Design review of the part built by this model. Coordinates are the model's own, in mm. A direction names the side the tool comes from. Coordinates: 2 decimals unless noted, no trailing zeros. Loops run counter-clockwise (first coordinate to the right, second up) from the corner with the lowest first, then second, coordinate; pieces in that order, holes last. Notation, with made-up numbers: (-16.5, 48.5) -> (20.5, 48.5) arc R29 cw to (20.5, 78.5) -> close; hole circle Ø5 at (-17, 28.25). An arc over 180 degrees is marked (long way). One line per item, written item: value. Start each with the question number.
1. Add section A-A on x = 38. Write out the cut boundary in (y, z), plus the area to 3 significant figures.
2. Add section C-C on x = 82.5. Write out the cut boundary in (y, z), plus the area to 3 significant figures.
3. Draft analysis for pull direction X (two halves, no side actions). For faces 5 (the flat face through (138.7, 24, 1)), 6 (the flat face through (46.24, 36, 2)), 7 (the flat face through (67, 24, 3)), state which applies: pulls with the +X half, pulls with the -X half, needs draft (parallel to the pull), parting line crosses it, or undercut.
4. For probe 1 along X at (y, z) = (13, 2.75); probe 2 along Y at (x, z) = (46, 0.25); probe 3 along X at (y, z) = (9, 2.35), list the stretches that pass through material, from the lowest coordinate up.
5. Insertion check: pin 1 (1.5 mm diameter, centred on x = 36, z = 1, fed in from -Y); pin 2 (0.9 mm diameter, centred on y = 13, z = 1.5, fed in from -X). Each pin has a flat end and moves straight along its axis. Give the tip position at first contact, or say it passes through.
6. Machinability: for faces 1 (the flat face through (100, 37.459, 2)), 2 (the flat face through (69, 8.959, 1)), 3 (the flat face through (-1, 33.959, 1)), 4 (the flat face through (-3, 27, 1)), which of the approach directions +Z, -Z, +X, -X, +Y, -Y give a long, thin tool a straight path to every point of the face, cutting with its end or side? Answer none if there is none.
7. Add section B-B on z = 0.9. Write out the cut boundary in (x, y), plus the area to 3 significant figures.
```python
from build123d import *

# Parameters (mm, degrees)
BOSS_EXTRUDE1_DEPTH = 3
SKETCH2_W           = 15
SKETCH2_H           = 3
CUT_EXTRUDE1_DEPTH  = 4


with BuildPart() as part:
    # Sketch1 → Boss-Extrude1 (new body)
    with BuildSketch(Plane.XY):
        with BuildLine():
            Line((138.7, 8.95909513), (138.7, 38.95909513))
            Line((138.7, 38.95909513), (0, 38.95909513))
            Line((0, 38.95909513), (0, 33.95909513))
            Line((0, 33.95909513), (-3, 33.95909513))
            Line((-3, 33.95909513), (-3, 18.95909513))
            Line((-3, 18.95909513), (0, 18.95909513))
            Line((0, 18.95909513), (0, 8.95909513))
            ThreePointArc((0, 8.95909513), (10, -1.04090487), (20, 8.95909513))
            Line((20, 8.95909513), (118.7, 8.95909513))
            ThreePointArc((118.7, 8.95909513), (128.7, -1.04090487), (138.7, 8.95909513))
        make_face()
    extrude(amount=BOSS_EXTRUDE1_DEPTH)

    # Sketch2 → Cut-Extrude1 (cut, through all)
    with BuildSketch(Plane.XY.offset(3)):
        with Locations((38.74, 35.95909513)):
            Rectangle(SKETCH2_W, SKETCH2_H)
        with Locations((99.97, 35.95909513)):
            Rectangle(SKETCH2_W, SKETCH2_H)
        with Locations((38.74, 11.95909513)):
            Rectangle(SKETCH2_W, SKETCH2_H)
        with Locations((99.97, 11.95909513)):
            Rectangle(SKETCH2_W, SKETCH2_H)
    extrude(amount=-CUT_EXTRUDE1_DEPTH, mode=Mode.SUBTRACT)


solid = part.part
```
Worked answers:
1. outline: (8.96, 0) -> (10.46, 0) -> (10.46, 3) -> (8.96, 3) -> close; (13.46, 0) -> (34.46, 0) -> (34.46, 3) -> (13.46, 3) -> close; (37.46, 0) -> (38.96, 0) -> (38.96, 3) -> (37.46, 3) -> close
1. area: 72.0 mm²
2. outline: (8.96, 0) -> (38.96, 0) -> (38.96, 3) -> (8.96, 3) -> close
2. area: 90.0 mm²
3. face 5: pulls with the +X half
3. face 6: undercut
3. face 7: needs draft
4. probe 1: x = 0 to 31.24, 46.24 to 92.47, 107.47 to 138.7
4. probe 2: y = 8.96 to 10.46, 13.46 to 34.46, 37.46 to 38.96
4. probe 3: x = 0 to 138.7
5. pin 1: stops at y = 8.96
5. pin 2: stops at x = 0
6. face 1: +Z, -Z
6. face 2: +Z, -Z, -Y
6. face 3: +Z, -Z, -X, +Y
6. face 4: +Z, -Z, -X, +Y, -Y
7. outline: (-3, 18.96) -> (0, 18.96) -> (0, 8.96) arc R10 ccw to (20, 8.96) -> (118.7, 8.96) arc R10 ccw to (138.7, 8.96) -> (138.7, 38.96) -> (0, 38.96) -> (0, 33.96) -> (-3, 33.96) -> close; hole (31.24, 10.46) -> (46.24, 10.46) -> (46.24, 13.46) -> (31.24, 13.46) -> close; hole (31.24, 34.46) -> (46.24, 34.46) -> (46.24, 37.46) -> (31.24, 37.46) -> close; hole (92.47, 10.46) -> (107.47, 10.46) -> (107.47, 13.46) -> (92.47, 13.46) -> close; hole (92.47, 34.46) -> (107.47, 34.46) -> (107.47, 37.46) -> (92.47, 37.46) -> close
7. area: 4,340 mm²
